from build123d import *

# Parameters (mm, degrees)
F1_DEPTH     = 6.096
F3_DEPTH     = 25.4
F4_T1_DEPTH  = 45.8630415712
F4_T3_DEPTH  = 24.3228960689
F4_T5_DEPTH  = 24.3228960689
F4_T8_ANGLE  = 50.429603728
F4_T10_ANGLE = 50.429603728
F4_T12_ANGLE = 50.429603728
F4_T14_ANGLE = 50.429603728


# Not quite as in the source:
# - a fillet or chamfer that OpenCascade refuses, or shapes differently, is made with other operations: its cross-section is extruded or revolved along the edge and cut away or added


with BuildPart() as f1:
    # F0 (on Front) → F1 (new body, symmetric)
    with BuildSketch(Plane.XZ):
        with BuildLine():
            Line((0, -39.7012000674), (8.9594220974, -32.2971154711))
            ThreePointArc((8.9594220974, -32.2971154711), (10.6592614203, -30.1074484367), (11.2643083058, -27.4022656866))
            Line((11.2643083058, -27.4022656866), (11.2643083058, 18.4607758846))
            ThreePointArc((11.2643083058, 18.4607758846), (10.6592614203, 21.1659586348), (8.9594220974, 23.3556256691))
            Line((8.9594220974, 23.3556256691), (0, 30.7597102655))
            ThreePointArc((0, 30.7597102655), (-5.4521439637, -4.470744901), (0, -39.7012000674))
        make_face()
    extrude(amount=F1_DEPTH, both=True)

    # F2 (on face) → F3 (cut)
    with BuildSketch(Plane.XZ.offset(6.096)):
        with BuildLine():
            ThreePointArc((5.8633539044, 18.8184664851), (5.322886305, 20.3627562227), (3.9373851632, 21.2329990657))
            ThreePointArc((3.9373851632, 21.2329990657), (3.3868539044, 18.8184664851), (2.8907187579, 16.3921725692))
            ThreePointArc((2.8907187579, 16.3921725692), (4.9527998741, 16.8999083103), (5.8633539044, 18.8184664851))
        make_face()
        with BuildLine():
            ThreePointArc((5.4685295173, -25.8524299357), (4.5748708681, -23.9477867911), (2.5388582003, -23.4177455604))
            ThreePointArc((2.5388582003, -23.4177455604), (2.9920295173, -25.8524299357), (3.4997963379, -28.2763162998))
            ThreePointArc((3.4997963379, -28.2763162998), (4.9143376067, -27.4137703405), (5.4685295173, -25.8524299357))
        make_face()
        with BuildLine():
            ThreePointArc((3.4997963379, -28.2763162998), (2.9920295173, -25.8524299357), (2.5388582003, -23.4177455604))
            ThreePointArc((2.5388582003, -23.4177455604), (0.5625907808, -26.3329293377), (3.4997963379, -28.2763162998))
        make_face()
        with BuildLine():
            ThreePointArc((3.3743560218, -4.470744901), (2.6588166523, -2.7294609185), (0.9256825651, -1.9944012387))
            ThreePointArc((0.9256825651, -1.9944012387), (0.8978560218, -4.470744901), (0.9256825651, -6.9470885632))
            ThreePointArc((0.9256825651, -6.9470885632), (2.6588166523, -6.2120288835), (3.3743560218, -4.470744901))
        make_face()
        with BuildLine():
            ThreePointArc((0.9256825651, -6.9470885632), (0.8978560218, -4.470744901), (0.9256825651, -1.9944012387))
            ThreePointArc((0.9256825651, -1.9944012387), (-1.5786439782, -4.470744901), (0.9256825651, -6.9470885632))
        make_face()
        with BuildLine():
            ThreePointArc((2.8907187579, 16.3921725692), (3.3868539044, 18.8184664851), (3.9373851632, 21.2329990657))
            ThreePointArc((3.9373851632, 21.2329990657), (0.9662878494, 19.3418327271), (2.8907187579, 16.3921725692))
        make_face()
    extrude(amount=-F3_DEPTH, mode=Mode.SUBTRACT)

    # F4: fillet of radius 5.08 on 10 edges, made by hand

    # F4_s2 → F4_t1 (cut)
    with BuildSketch(Plane.XY.offset(-27.4022656866)):
        with BuildLine():
            ThreePointArc((6.1843083058, -6.096), (9.7764107542, -4.6081024484), (11.2643083058, -1.016))
            Line((11.2643083058, -1.016), (11.2643083058, -6.096))
            Line((11.2643083058, -6.096), (6.1843083058, -6.096))
        make_face()
        with BuildLine():
            ThreePointArc((6.1843083058, 6.096), (9.7764107542, 4.6081024484), (11.2643083058, 1.016))
            Line((11.2643083058, 1.016), (11.2643083058, 6.096))
            Line((11.2643083058, 6.096), (6.1843083058, 6.096))
        make_face()
    extrude(amount=F4_T1_DEPTH, mode=Mode.SUBTRACT)

    # F4_s4 → F4_t3 (cut)
    with BuildSketch(Plane(origin=(-29.284836754, 0, -24.2010485008), x_dir=(0, 1, 0), z_dir=(0.7708424857, 0, 0.637025794))):
        with BuildLine():
            ThreePointArc((1.016, -30.6033717472), (4.6081024484, -29.1154741956), (6.096, -25.5233717472))
            Line((6.096, -25.5233717472), (6.096, -30.6033717472))
            Line((6.096, -30.6033717472), (1.016, -30.6033717472))
        make_face()
        with BuildLine():
            ThreePointArc((-1.016, -30.6033717472), (-4.6081024484, -29.1154741956), (-6.096, -25.5233717472))
            Line((-6.096, -25.5233717472), (-6.096, -30.6033717472))
            Line((-6.096, -30.6033717472), (-1.016, -30.6033717472))
        make_face()
    extrude(amount=F4_T3_DEPTH, mode=Mode.SUBTRACT)

    # F4_s6 → F4_t5 (cut)
    with BuildSketch(Plane(origin=(-6.1450273998, 0, 5.078263109), x_dir=(0, 1, 0), z_dir=(-0.7708424857, 0, 0.637025794))):
        with BuildLine():
            ThreePointArc((6.096, -18.630891522), (4.6081024484, -22.2229939704), (1.016, -23.710891522))
            Line((1.016, -23.710891522), (6.096, -23.710891522))
            Line((6.096, -23.710891522), (6.096, -18.630891522))
        make_face()
        with BuildLine():
            ThreePointArc((-6.096, -18.630891522), (-4.6081024484, -22.2229939704), (-1.016, -23.710891522))
            Line((-1.016, -23.710891522), (-6.096, -23.710891522))
            Line((-6.096, -23.710891522), (-6.096, -18.630891522))
        make_face()
    extrude(amount=F4_T5_DEPTH, mode=Mode.SUBTRACT)

    # F4_s7 → F4_t8 (revolve, cut)
    with BuildSketch(Plane(origin=(-10.5357150876, 0, -8.7067363212), x_dir=(0, 1, 0), z_dir=(-0.7708424857, 0, -0.637025794))):
        with BuildLine():
            ThreePointArc((6.096, 25.5233717472), (4.6081024484, 29.1154741956), (1.016, 30.6033717472))
            Line((1.016, 30.6033717472), (6.096, 30.6033717472))
            Line((6.096, 30.6033717472), (6.096, 25.5233717472))
        make_face()
    revolve(axis=Axis((4.9143083058, 6.096, -27.4022656866), (0, -1, 0)), revolution_arc=F4_T8_ANGLE, mode=Mode.SUBTRACT)

    # F4_s9 → F4_t10 (revolve, cut)
    with BuildSketch(Plane.XY.offset(18.4607758846)):
        with BuildLine():
            ThreePointArc((6.1843083058, 6.096), (9.7764107542, 4.6081024484), (11.2643083058, 1.016))
            Line((11.2643083058, 1.016), (11.2643083058, 6.096))
            Line((11.2643083058, 6.096), (6.1843083058, 6.096))
        make_face()
    revolve(axis=Axis((4.9143083058, 6.096, 18.4607758846), (0, -1, 0)), revolution_arc=F4_T10_ANGLE, mode=Mode.SUBTRACT)

    # F4_s11 → F4_t12 (revolve, cut)
    with BuildSketch(Plane(origin=(-10.5357150876, 0, -8.7067363212), x_dir=(0, 1, 0), z_dir=(-0.7708424857, 0, -0.637025794))):
        with BuildLine():
            ThreePointArc((-1.016, 30.6033717472), (-4.6081024484, 29.1154741956), (-6.096, 25.5233717472))
            Line((-6.096, 25.5233717472), (-6.096, 30.6033717472))
            Line((-6.096, 30.6033717472), (-1.016, 30.6033717472))
        make_face()
    revolve(axis=Axis((4.9143083058, -6.096, -27.4022656866), (0, -1, 0)), revolution_arc=F4_T12_ANGLE, mode=Mode.SUBTRACT)

    # F4_s13 → F4_t14 (revolve, cut)
    with BuildSketch(Plane.XY.offset(18.4607758846)):
        with BuildLine():
            ThreePointArc((6.1843083058, -6.096), (9.7764107542, -4.6081024484), (11.2643083058, -1.016))
            Line((11.2643083058, -1.016), (11.2643083058, -6.096))
            Line((11.2643083058, -6.096), (6.1843083058, -6.096))
        make_face()
    revolve(axis=Axis((4.9143083058, -6.096, 18.4607758846), (0, -1, 0)), revolution_arc=F4_T14_ANGLE, mode=Mode.SUBTRACT)


solid = f1.part
Read the model definition and answer for the solid it produces. Units are mm, in the model's axes. Coordinates: 2 decimals unless noted, no trailing zeros. Write each loop counter-clockwise with the first axis right and the second up, starting at its lowest first coordinate (ties: lowest second). Pieces come first, ordered by that corner, then holes. Notation, with made-up numbers: M -3,11 L 28,11 A30 cw 28,43 Z; hole C -21.5,32 d10. An arc over 180 degrees is marked long. Use a Markdown table: item, result.
Q1. The part is cut by section B-B, the plane z = -15. Write down the section's boundary in (x, y), then the cut area to 3 significant figures.
Answer block:
| item | result |
|---|---|
| outline | M -4.98,-6.1 L 6.18,-6.1 A5.08 ccw 11.26,-1.02 L 11.26,1.02 A5.08 ccw 6.18,6.1 L -4.98,6.1 Z |
| area | 187 mm2 |
Q2. Straight lines are drawn through the part: L1, parallel to Z at x = 4.25, y = -2.5; L2, parallel to Z at x = 5, y = -0.5; L3, parallel to X at y = 3, z = -3. For each, find the intervals that lie inside material, in ascending order. Write a range as [from, to].
Answer block:
| item | result |
|---|---|
| L1 | z = [-35.9, -27.99], [-23.72, 16.5], [21.14, 26.96] |
| L2 | z = [-35.57, -27.3], [-24.4, 16.94], [20.7, 26.63] |
| L3 | x = [-5.44, -1.09], [2.89, 10.86] |
Q3. The part is cut by section A-A, the plane y = -0.25. Write down the section's boundary in (x, z), then the cut area to 3 significant figures.
Answer block:
| item | result |
|---|---|
| outline | M 0,-39.7 L 8.96,-32.3 A6.35 ccw 11.26,-27.4 L 11.26,18.46 A6.35 ccw 8.96,23.36 L 0,30.76 A116.55 ccw Z; hole C 0.9,-4.47 d4.95; hole C 2.99,-25.85 d4.95; hole C 3.39,18.82 d4.95 |
| area | 886 mm2 |
Q4. The part is cut by section C-C, the plane y = 4.75. Give the number of separate pieces and of enclosed holes in the cut face, then the cut area to 3 significant figures.
Answer block:
| item | result |
|---|---|
| separate pieces | 1 |
| enclosed holes | 3 |
| area | 758 mm2 |
Q5. Each of these flat-tipped pins is pushed along its axis until it touches: pin 1 Ø1 at (x, y) = (6.5, -3.5) entering from -Z; pin 2 Ø1 at (y, z) = (2.5, -13) entering from +X; pin 3 Ø3 at (x, y) = (9.5, -1.5) entering from +Z. Where does it stop, or does it pass through?
Answer block:
| item | result |
|---|---|
| pin 1 | stops at z = -34.02 |
| pin 2 | stops at x = 11.17 |
| pin 3 | stops at z = 24.13 |
Q6. The part is cut by section D-D, the plane z = 9. Write down the section's boundary in (x, y).
Answer block:
| item | result |
|---|---|
| outline | M -4.67,-6.1 L 6.18,-6.1 A5.08 ccw 11.26,-1.02 L 11.26,1.02 A5.08 ccw 6.18,6.1 L -4.67,6.1 Z |
